For this review, take the finished solid that the model builds, in its own axes (mm). A direction names the side the tool comes from. Coordinates: 2 decimals unless noted, no trailing zeros. Loops run counter-clockwise (first coordinate to the right, second up) from the corner with the lowest first, then second, coordinate; pieces in that order, holes last. Notation, with made-up numbers: (31.5, 15) -> (90.5, 15) arc R34 cw to (90.5, 47) -> close; hole circle Ø3 at (10, -5). An arc over 180 degrees is marked (long way). One line per item, written item: value.
from build123d import *

# Parameters (mm, degrees)
SKETCH1_W           = 195
SKETCH1_H           = 136
SKETCH1_W_2         = 171
SKETCH1_H_2         = 112
SKETCH1_W_3         = 160
SKETCH1_H_3         = 96
SKETCH1_W_4         = 29
SKETCH1_H_4         = 3
BOSS_EXTRUDE1_DEPTH = 2
SKETCH1_3_W         = 195
SKETCH1_3_H         = 136
SKETCH1_3_W_2       = 171
SKETCH1_3_H_2       = 112
SKETCH1_3_W_3       = 160
SKETCH1_3_H_3       = 96
SKETCH1_3_W_4       = 29
SKETCH1_3_H_4       = 3
BOSS_EXTRUDE2_DEPTH = 2
SKETCH2_R           = 3.175
SKETCH2_R_2         = 3.673722566
CUT_EXTRUDE1_DEPTH  = 2.794


with BuildPart() as part:
    # Sketch1 → Boss-Extrude1 (new body)
    # profile 1 of 3: a face of its own
    with BuildSketch(Plane.XY):
        Rectangle(SKETCH1_W, SKETCH1_H)
        Polygon((85.5, 56), (85.5, -56), (14.5, -56), (14.5, -59), (-14.5, -59), (-14.5, -56), (-85.5, -56), (-85.5, 56), align=None, mode=Mode.SUBTRACT)
    # profile 2 of 3: a face of its own
    with BuildSketch(Plane.XY):
        Rectangle(SKETCH1_W_2, SKETCH1_H_2)
        with Locations((0, 3)):
            Rectangle(SKETCH1_W_3, SKETCH1_H_3, mode=Mode.SUBTRACT)
    # profile 3 of 3: a face of its own
    with BuildSketch(Plane.XY):
        with Locations((0, -57.5)):
            Rectangle(SKETCH1_W_4, SKETCH1_H_4)
    extrude(amount=-BOSS_EXTRUDE1_DEPTH)

    # Sketch1_3 → Boss-Extrude2 (add)
    # profile 1 of 3: a face of its own
    with BuildSketch(Plane.XY):
        Rectangle(SKETCH1_3_W, SKETCH1_3_H)
        Polygon((85.5, 56), (85.5, -56), (14.5, -56), (14.5, -59), (-14.5, -59), (-14.5, -56), (-85.5, -56), (-85.5, 56), align=None, mode=Mode.SUBTRACT)
    # profile 2 of 3: a face of its own
    with BuildSketch(Plane.XY):
        Rectangle(SKETCH1_3_W_2, SKETCH1_3_H_2)
        with Locations((0, 3)):
            Rectangle(SKETCH1_3_W_3, SKETCH1_3_H_3, mode=Mode.SUBTRACT)
    # profile 3 of 3: a face of its own
    with BuildSketch(Plane.XY):
        with Locations((0, -57.5)):
            Rectangle(SKETCH1_3_W_4, SKETCH1_3_H_4)
    extrude(amount=BOSS_EXTRUDE2_DEPTH)

    # Sketch2 → Cut-Extrude1 (cut)
    with BuildSketch(Plane.XY.offset(2)):
        with Locations((-90.5, 61)):
            Circle(SKETCH2_R)
        with Locations((90.5, 61)):
            Circle(SKETCH2_R)
        with Locations((90.5, -61)):
            Circle(SKETCH2_R)
        with Locations((-90.5, -61)):
            Circle(SKETCH2_R)
        with Locations((-30.166666667, -61)):
            Circle(SKETCH2_R)
        with Locations((30.166666667, -61)):
            Circle(SKETCH2_R)
        with Locations((90.5, 0)):
            Circle(SKETCH2_R_2)
        with Locations((-30.166666667, 61)):
            Circle(SKETCH2_R)
        with Locations((30.166666667, 61)):
            Circle(SKETCH2_R)
        with Locations((-90.5, 0)):
            Circle(SKETCH2_R_2)
    extrude(amount=-CUT_EXTRUDE1_DEPTH, mode=Mode.SUBTRACT)


solid = part.part
1. Insertion check: pin 1 Ø1.9 at (x, y) = (-89, 61.5) entering from +Z. The pin has a flat end and moves straight along its axis. Give the tip position at first contact, or say it passes through.
Return value:
pin 1: stops at z = -0.79
2. Take a section at A-A, the plane y = 0. Give the boundary of the cut face in (x, z).
Return value:
outline: (-97.5, -2) -> (-80, -2) -> (-80, 2) -> (-86.83, 2) -> (-86.83, -0.79) -> (-94.17, -0.79) -> (-94.17, 2) -> (-97.5, 2) -> close; (80, -2) -> (97.5, -2) -> (97.5, 2) -> (94.17, 2) -> (94.17, -0.79) -> (86.83, -0.79) -> (86.83, 2) -> (80, 2) -> close
3. Take a section at C-C, the plane z = 0.95. Give the number of separate pieces and of enclosed holes in the cut face, and give its area (3 significant figures).
Return value:
separate pieces: 1
enclosed holes: 11
area: 10,800 mm2
4. Take a section at D-D, the plane y = -61. Give the boundary of the cut face in (x, z) (3 decimals).
Return value:
outline: (-97.5, -2) -> (97.5, -2) -> (97.5, 2) -> (93.675, 2) -> (93.675, -0.794) -> (87.325, -0.794) -> (87.325, 2) -> (33.342, 2) -> (33.342, -0.794) -> (26.992, -0.794) -> (26.992, 2) -> (-26.992, 2) -> (-26.992, -0.794) -> (-33.342, -0.794) -> (-33.342, 2) -> (-87.325, 2) -> (-87.325, -0.794) -> (-93.675, -0.794) -> (-93.675, 2) -> (-97.5, 2) -> close
5. The part is to be moulded in two halves that separate along X. For faces 4 (the flat face through (14, -50, 2)), 5 (the flat face through (97.5, -1, 0)), 6 (the cylindrical face through (-87.106, -1.407, 0.623)), say which applies: pulls with the +X half, pulls with the -X half, needs draft (parallel to the pull), parting line crosses it, or undercut.
Return value:
face 4: needs draft
face 5: pulls with the +X half
face 6: undercut
6. To check wall thickness, follow probe 1 along Y at (x, z) = (90.5, -0.05) (3 decimals); probe 2 along X at (y, z) = (-39.5, -0.5); probe 3 along Y at (x, z) = (29.5, -1.3). State the ranges of each line that lie inside material, in increasing order. Write a range as from..to.
Return value:
probe 1: y = -68..-64.175, -57.825..-3.674, 3.674..57.825, 64.175..68
probe 2: x = -97.5..-80, 80..97.5
probe 3: y = -68..-45, 51..68
7. For faces 1 (the cylindrical face through (93.894, -1.407, 0.623)), 2 (the flat face through (-80, 2, 0)), 3 (the flat face through (-1, -68, 0)), list the 3-axis set-ups (+Z, -Z, +X, -X, +Y, -Y) from which the entire face can be reached by the end or side of a thin tool; tool diameter is ignored.
Return value:
face 1: +Z
face 2: +Z, -Z
face 3: +Z, -Z, +X, -X, -Y
8. Take a section at B-B, the plane x = -50. Give the boundary of the cut face in (y, z), and give its area (3 significant figures).
Return value:
outline: (-68, -2) -> (-45, -2) -> (-45, 2) -> (-68, 2) -> close; (51, -2) -> (68, -2) -> (68, 2) -> (51, 2) -> close
area: 160 mm2
